Build history of the part. All positions in model axes, mm. Face numbers are marked on the shaded views. Coordinates: 2 decimals unless noted, no trailing zeros. Order: outer loops, then holes, each group sorted by start corner. A loop starts at its lowest first (then second) coordinate and runs counter-clockwise, first axis right, second up. Notation, with made-up numbers: (-21, -28.5) - (31, -28.5) arc R9 cw to (31, -21.5) - close; hole circle Ø1 at (81.5, 89.25). An arc over 180 degrees is marked (long way). Return JSON: item names as keys, results as strings.
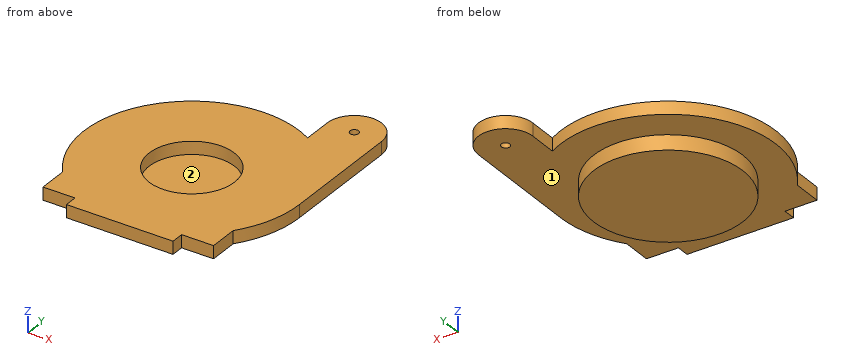
from build123d import *

# Parameters (mm, degrees)
SKETCH1_R           = 17.265633628
SKETCH1_R_2         = 1
SKETCH1_R_3         = 10
SKETCH1_W           = 25
SKETCH1_H           = 3
BOSS_EXTRUDE5_DEPTH = 3
SKETCH2_R           = 17.5
BOSS_EXTRUDE6_DEPTH = 3.5


with BuildPart() as part:
    # Sketch1 → Boss-Extrude5 (new body)
    # profile 1 of 3: a face of its own
    with BuildSketch(Plane.XY):
        with BuildLine():
            Line((0, 0), (7.5, 0))
            Line((7.5, 0), (32.5, 0))
            Line((32.5, 0), (40, 0))
            Line((40, 0), (40, 6.867081787))
            ThreePointArc((40, 6.867081787), (43.887871625, 14.125845764), (45.231531638, 22.249870507))
            Line((45.231531638, 22.249870507), (45.231531638, 51.023857348))
            ThreePointArc((45.231531638, 51.023857348), (38.865765819, 57.389623167), (32.5, 51.023857348))
            Line((32.5, 51.023857348), (32.5, 44.167447672))
            ThreePointArc((32.5, 44.167447672), (0.97654543, 38.82510399), (0, 6.867081787))
            Line((0, 6.867081787), (0, 0))
        make_face()
        with Locations((20, 22.249870507)):
            Circle(SKETCH1_R, mode=Mode.SUBTRACT)
        with Locations((38.865765819, 51.023857348)):
            Circle(SKETCH1_R_2, mode=Mode.SUBTRACT)
    # profile 2 of 3: a face of its own
    with BuildSketch(Plane.XY):
        with Locations((20, 22.249870507)):
            Circle(SKETCH1_R)
        with Locations((20, 22.249870507)):
            Circle(SKETCH1_R_3, mode=Mode.SUBTRACT)
    # profile 3 of 3: a face of its own
    with BuildSketch(Plane.XY):
        with Locations((20, -1.5)):
            Rectangle(SKETCH1_W, SKETCH1_H)
    extrude(amount=BOSS_EXTRUDE5_DEPTH)

    # Sketch2 → Boss-Extrude6 (add)
    with BuildSketch(Plane(origin=(0, 0, 0), x_dir=(-1, 0, 0), z_dir=(0, 0, -1))):
        with Locations(Location((-20, 22.249870507, 0), (0, 0, 180))):
            Circle(SKETCH2_R)
    extrude(amount=BOSS_EXTRUDE6_DEPTH)


solid = part.part
1. Drop flat-ended pins along their axis: pin 1 (2.5 mm diameter, centred on x = 5.5, z = 2, fed in from -Y); pin 2 (1.5 mm diameter, centred on x = 20.5, z = -0.5, fed in from +Y); pin 3 (0.9 mm diameter, centred on y = -1.5, z = 1, fed in from +X). Give the stop position or say it passes through.
Check values:
{"pin 1": "y = 0", "pin 2": "y = 47.48", "pin 3": "x = 32.5"}
2. Cut at A-A on z = 2.25. Give the cut face in (x, y).
Check values:
{"outline": "(0, 0) - (7.5, 0) - (7.5, -3) - (32.5, -3) - (32.5, 0) - (40, 0) - (40, 6.87) arc R25.23 ccw to (45.23, 22.25) - (45.23, 51.02) arc R6.37 ccw to (32.5, 51.02) - (32.5, 44.17) arc R25.23 ccw to (0, 6.87) - close; hole circle Ø20 at (20, 22.25); hole circle Ø2 at (38.87, 51.02)"}
3. Cut at C-C on y = 15. Give the cut face in (x, z).
Check values:
{"outline": "(-4.17, 0) - (4.07, 0) - (4.07, -3.5) - (35.93, -3.5) - (35.93, 0) - (44.17, 0) - (44.17, 3) - (26.89, 3) - (26.89, 0) - (13.11, 0) - (13.11, 3) - (-4.17, 3) - close"}
4. Cut at B-B on x = 20. Give the cut face in (y, z).
Check values:
{"outline": "(-3, 0) - (4.75, 0) - (4.75, -3.5) - (39.75, -3.5) - (39.75, 0) - (47.48, 0) - (47.48, 3) - (32.25, 3) - (32.25, 0) - (12.25, 0) - (12.25, 3) - (-3, 3) - close"}
5. Mould opens along Y. For the marked faces 1 and 2 say: pulls with the +Y half, pulls with the -Y half, needs draft (parallel to the pull), parting line crosses it, or undercut.
Check values:
{"face 1": "needs draft", "face 2": "undercut"}
6. Cut at D-D on x = 33.5. Give the cut face in (y, z).
Check values:
{"outline": "(0, 0) - (11.11, 0) - (11.11, -3.5) - (33.39, -3.5) - (33.39, 0) - (54.45, 0) - (54.45, 3) - (0, 3) - close"}
7. Probe L1, parallel to Y at x = 20, z = 0.25; L2, parallel to X at y = 51, z = 1; L3, parallel to Z at x = 40.5, y = 38. List the from-to ranges inside material, lowest first.
Check values:
{"L1": "-3 to 12.25, 32.25 to 47.48", "L2": "32.5 to 37.87, 39.87 to 45.23", "L3": "0 to 3"}
